Could you check a few things on this model? Use its own coordinates, in mm. Coordinates: 2 decimals unless noted, no trailing zeros. Write each loop counter-clockwise with the first axis right and the second up, starting at its lowest first coordinate (ties: lowest second). Pieces come first, ordered by that corner, then holes.
Item 1: For P1, Ø2, axis at x = 0.37, y = 17.7, coming from the -Z side, with a flat end and sliding along its axis, tell me the tip position at first contact or that it passes through.
Item 2: If I drill on probe 1 along Y at (x, z) = (0.25, 1.85); probe 2 along Y at (x, z) = (1, 1.8); probe 3 along X at (y, z) = (18, 0.5), over which ranges is the centre line in solid material (lowest first)?
Item 3: I want a section at B-B on x = -5. Please give me the cut outline in (y, z).
Item 4: I want a section at C-C on x = 8.5. Please give me the cut outline in (y, z).
Item 5: I want a section at A-A on z = 1.1. Please give me the cut outline in (x, y).
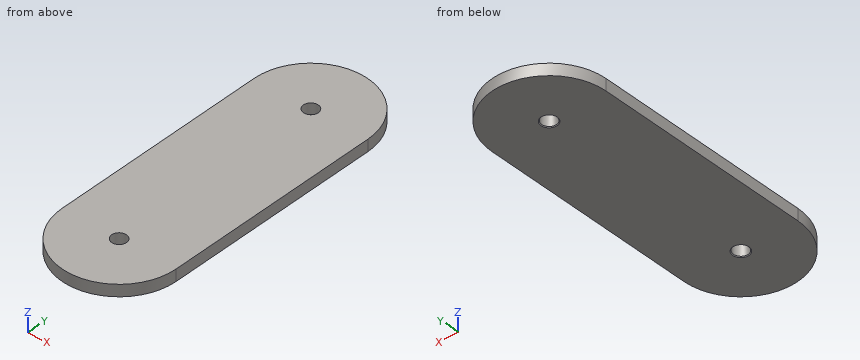
Autodesk Fusion 360 part; units mm, degrees
sketch "Sketch1" plane through (0, 0, 0) normal (0, 0, 1) x (1, 0, 0)
  line L0 (-9.3846, 17.702) -> (-9.3846, -19.298)
  arc A0 (-9.3846, -19.298) -> (10.1154, -19.298) centre (0.3654, -19.298) ccw
  line L1 (10.1154, -19.298) -> (10.1154, 17.702)
  arc A1 (10.1154, 17.702) -> (-9.3846, 17.702) centre (0.3654, 17.702) ccw
  line L2 (0.3654, 17.702) -> (0.3654, -19.298) construction
  dimension "d1" = 37
  dimension "d2" = 9.75
extrude "Extrude1" add sketch "Sketch1" along normal blind 2
hole "Hole1" at (0.3654, 17.702, 0) at (0.3654, -19.298, 0) direction (0, 0, 1) diameter 2.529 depth 2 tip angle 180 countersink diameter 2.782 countersink angle 90
Response values:
1. P1: passes through
2. probe 1: y = -29.05 to -20.56, -18.04 to 16.44, 18.96 to 27.45
2. probe 2: y = -29.03 to -20.39, -18.2 to 16.61, 18.8 to 27.43
2. probe 3: x = -9.38 to -0.86, 1.59 to 10.11
3. outline: (-27.44, 0) - (25.84, 0) - (25.84, 2) - (-27.44, 2) - close
4. outline: (-24.67, 0) - (23.08, 0) - (23.08, 2) - (-24.67, 2) - close
5. outline: (-9.38, -19.3) arc R9.75 ccw to (10.12, -19.3) - (10.12, 17.7) arc R9.75 ccw to (-9.38, 17.7) - close; hole circle Ø2.53 at (0.37, -19.3); hole circle Ø2.53 at (0.37, 17.7)
